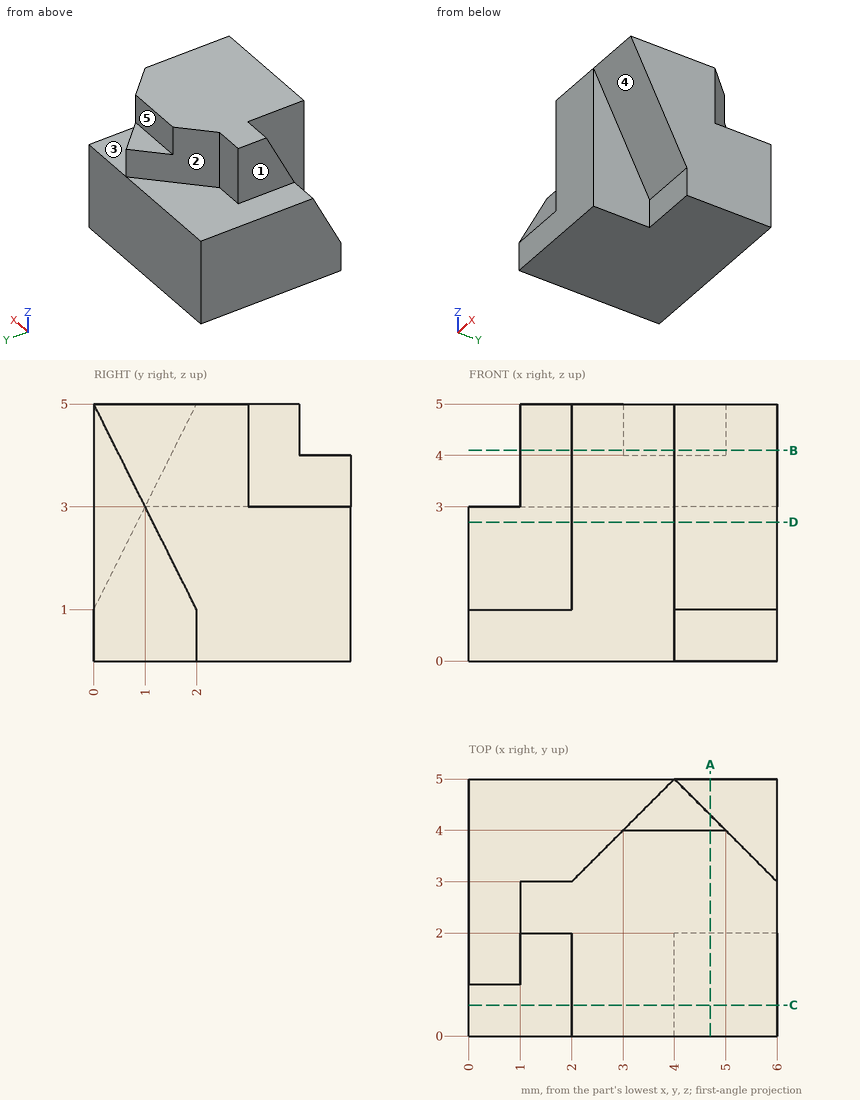
For this review, use the dimensioned drawing (mm, ordinates from the lowest corner) and the shaded views. A direction names the side the tool comes from. Coordinates: 2 decimals unless noted, no trailing zeros. Write each loop counter-clockwise with the first axis right and the second up, starting at its lowest first coordinate (ties: lowest second). Pieces come first, ordered by that corner, then holes. Notation, with made-up numbers: (34, -40) -> (38, -40) arc R30 ccw to (38, -6) -> close; hole circle Ø11 at (34.25, 12). An arc over 180 degrees is marked (long way). Write each question's results on one line, items separated by ' | '. Start each with the question number.
(1) Clearance check with flat-ended pins moving along their axes: P1, Ø0.8, axis at x = 4, z = 4.5, coming from the +Y side; P2, Ø0.6, axis at y = 2, z = 4.5, coming from the -X side; P3, Ø1.1, axis at x = 5, z = 0.5, coming from the -Y side (3 decimals). State where each tip first meets the part, or that it passes through.
(2) Take a section at A-A on x = 4.7. Write out the cut boundary in (y, z).
(3) Tool access review of the marked faces 1, 2, 3, 4 and 5: name each direction out of +Z, -Z, +X, -X, +Y, -Y from which nothing blocks a thin tool from reaching the whole face with its end or side.
(4) For line 1 along Z through (x, y) = (0.85, 3.6); line 2 along X through (y, z) = (0.8, 1.6); line 3 along Y through (x, z) = (4.05, 0.45), list the stretches that pass through material, from the lowest coordinate up. Write a range as from..to.
(5) Take a section at B-B on z = 4.1. Write out the cut boundary in (x, y), and give its area (4 significant figures).
(6) Take a section at C-C on y = 0.6. Write out the cut boundary in (x, z), and give its area (3 significant figures).
(7) Take a section at D-D on z = 2.7. Write out the cut boundary in (x, y), and give its area (3 significant figures).
Results found:
1) P1: stops at y = 4 | P2: stops at x = 1 | P3: stops at y = 1.975
2) outline: (0, 5) -> (2, 1) -> (2, 0) -> (5, 0) -> (5, 3) -> (4.3, 3) -> (4.3, 4) -> (4, 4) -> (4, 5) -> close
3) face 1: +Z, -X, +Y, -Y | face 2: +Z, -X, +Y | face 3: +Z, +X, +Y | face 4: -Z, +X, -Y | face 5: +Z, +X, -X, +Y
4) line 1: z = 0..3 | line 2: x = 0..4 | line 3: y = 2..5
5) outline: (1, 1.55) -> (2, 1.55) -> (2, 0) -> (4, 0) -> (4, 0.45) -> (6, 0.45) -> (6, 3) -> (5, 4) -> (3, 4) -> (2, 3) -> (1, 3) -> close | area: 15.55 mm2
6) outline: (0, 0) -> (4, 0) -> (4, 3.8) -> (6, 3.8) -> (6, 5) -> (2, 5) -> (2, 2.2) -> (0, 2.2) -> close | area: 16.8 mm2
7) outline: (0, 0.85) -> (2, 0.85) -> (2, 0) -> (4, 0) -> (4, 1.15) -> (6, 1.15) -> (6, 5) -> (0, 5) -> close | area: 26.0 mm2
